Verification items for this drawing (mm, ordinates from the low corner). Round coordinates to 2 decimals unless told otherwise and drop trailing zeros. Loops run counter-clockwise (first coordinate to the right, second up) from the corner with the lowest first, then second, coordinate; pieces in that order, holes last. Notation, with made-up numbers: M -12.75,-24 L 42.25,-24 A10 cw 42.25,-11 Z; hole C 58,19 d4. An arc over 180 degrees is marked long. One line per item, written item: value.
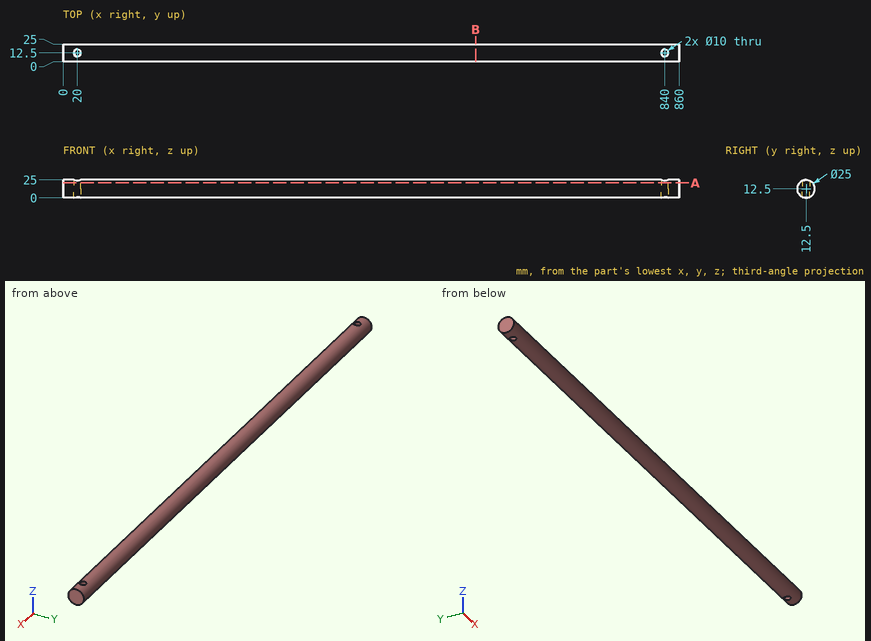
(1) Sectioned sample at B-B on x = 576. Enter the section's corners in (y, z), and give its area (3 significant figures).
Completed:
outline: C 12.5,12.5 d25
area: 491 mm^2
(2) Thickness scan on L1, parallel to Z at x = 406, y = 11; L2, parallel to Z at x = 390.5, y = 1. Record the ranges inside material, lowest first. Write a range as from..to.
Completed:
L1: z = 0.09..24.91
L2: z = 7.6..17.4
(3) Sectioned sample at A-A on z = 21. Enter the section's corners in (x, y).
Completed:
outline: M 0,3.33 L 860,3.33 L 860,21.67 L 0,21.67 Z; hole C 20,12.5 d10; hole C 840,12.5 d10
(4) Depth check by flat-ended pin: pin 1 Ø1 at (x, z) = (95, 5) entering from -Y; pin 2 Ø1 at (x, y) = (545, 8.5) entering from +Z; pin 3 Ø6 at (x, y) = (20, 12.5) entering from -Z; pin 4 Ø6 at (x, y) = (526, 20.5) entering from -Z. Enter the tip coordinate at first touch or a pass-through.
Completed:
pin 1: stops at y = 2.14
pin 2: stops at z = 24.5
pin 3: passes through
pin 4: stops at z = 1.04
